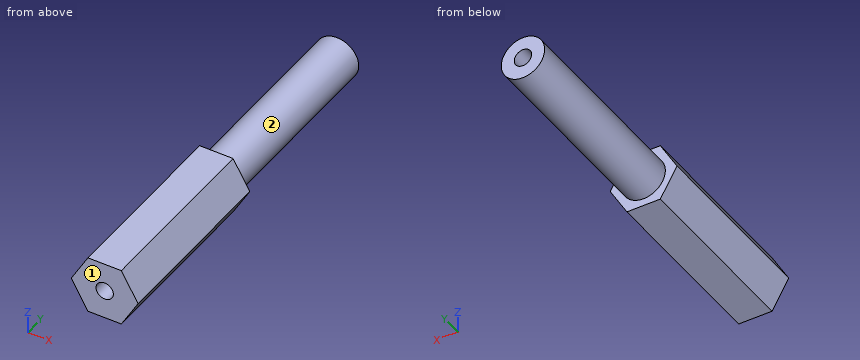
Autodesk Inventor part; units mm, degrees
ref_plane "YZ Plane" through (0, 0, 0) normal (1, 0, 0) x (0, 1, 0)
ref_plane "XZ Plane" through (0, 0, 0) normal (0, 1, 0) x (-1, 0, 0)
ref_plane "XY Plane" through (0, 0, 0) normal (0, 0, 1) x (1, 0, 0)
sketch "Sketch1" plane through (0, 0, 0) normal (0, 1, 0) x (-1, 0, 0)
  line L0 (3.6662, -6.35) -> (-3.6662, -6.35)
  line L1 (-3.6662, -6.35) -> (-7.3323, 0)
  line L2 (-7.3323, 0) -> (-3.6662, 6.35)
  line L3 (-3.6662, 6.35) -> (3.6662, 6.35)
  line L4 (3.6662, 6.35) -> (7.3323, 0)
  line L5 (7.3323, 0) -> (3.6662, -6.35)
  point P0 (0, 0)
  point P1 (0, 0)
  dimension "d0" = 12.7
extrude "Extrusion1" add sketch "Sketch1" against normal blind 39.6875
sketch "Sketch2" plane through (0, 0, 0) normal (0, 1, 0) x (1, 0, 0)
  circle A0 centre (0, 0) radius 4.7625
  dimension "d3" = 9.525
extrude "Extrusion2" add sketch "Sketch2" along normal blind 42.8625
sketch "Sketch3" plane through (0, -39.6875, 0) normal (0, -1, 0) x (1, 0, 0)
  circle A0 centre (0, 0) radius 4.7625
  circle A1 centre (0, 0) radius 1.905
  dimension "d7" = 3.81
extrude "Extrusion3" cut sketch "Sketch3" against normal blind 25.4 contours A1
sketch "Sketch4" plane through (0, 42.8625, 0) normal (0, 1, 0) x (1, 0, 0)
  circle A0 centre (0, 0) radius 1.905
extrude "Extrusion4" cut sketch "Sketch4" against normal blind 25.4
properties part number "Roller driven shaft" material "Aluminum 6061"
Work out the finished part from the listing and answer in its coordinate system (mm). Face numbers are marked on the shaded views. A direction names the side the tool comes from. Give positions to 0.01 mm unless a question says otherwise; leave off trailing zeros. Write each loop counter-clockwise with the first axis right and the second up, starting at its lowest first coordinate (ties: lowest second). Pieces come first, ordered by that corner, then holes. Notation, with made-up numbers: M -19,2.25 L 35,2.25 A28 ccw 35,23.25 Z; hole C -25.75,62.5 d7. An arc over 180 degrees is marked long. Answer as CSV lines item,"result".
Q1. Find the intervals of material crossed by probe 1 along Z at (x, y) = (0, 33.25) (1 decimal); probe 2 along Z at (x, y) = (0, -31.5) (3 decimals), in increasing order. Write a range as [from, to].
A:
probe 1,"z = [-4.8, -1.9], [1.9, 4.8]"
probe 2,"z = [-6.35, -1.905], [1.905, 6.35]"
Q2. Given P1, Ø6, axis at y = 12, z = -3.5, coming from the -X side; P2, Ø2, axis at y = 26, z = 0.5, coming from the +X side; P3, Ø3.5, axis at x = 0, z = 0, coming from the -Y side, each flat-ended and moving along its own axis, determine where each tip first touches the part or whether it passes through.
A:
P1,"stops at x = -4.74"
P2,"stops at x = 4.76"
P3,"stops at y = -14.29"
Q3. A cutting plane is placed at A-A on y = -28.5. Write down the section's boundary in (x, z) (3 decimals), plus the area to 3 significant figures.
A:
outline,"M -7.332,0 L -3.666,-6.35 L 3.666,-6.35 L 7.332,0 L 3.666,6.35 L -3.666,6.35 Z; hole C 0,0 d3.81"
area,"128 mm²"
Q4. A tool of negligible diameter and unlimited length cuts with its end or side. For the marked faces 1 and 2, from which of +Z, -Z, +X, -X, +Y, -Y can it reach the whole face along a straight path? Write none if from no direction.
A:
face 1,"+Z, -Z, +X, -X, -Y"
face 2,"+Y"
Q5. A cutting plane is placed at D-D on y = -2. Write down the section's boundary in (x, z), plus the area to 3 significant figures.
A:
outline,"M -7.33,0 L -3.67,-6.35 L 3.67,-6.35 L 7.33,0 L 3.67,6.35 L -3.67,6.35 Z"
area,"140 mm²"
Q6. A cutting plane is placed at C-C on z = -0.75. Write down the section's boundary in (x, y), plus the area to 3 significant figures.
A:
outline,"M -6.9,-39.69 L -1.75,-39.69 L -1.75,-14.29 L 1.75,-14.29 L 1.75,-39.69 L 6.9,-39.69 L 6.9,0 L 4.7,0 L 4.7,42.86 L 1.75,42.86 L 1.75,17.46 L -1.75,17.46 L -1.75,42.86 L -4.7,42.86 L -4.7,0 L -6.9,0 Z"
area,"773 mm²"
